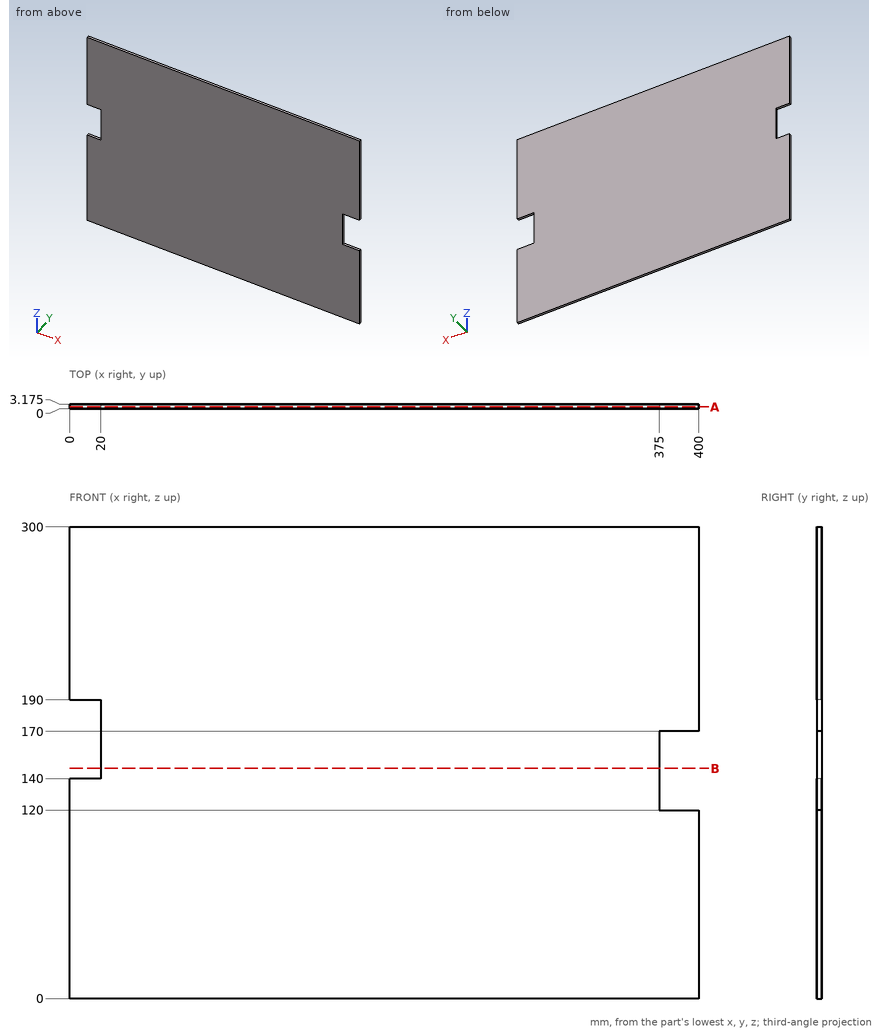
Source: three-view drawing plus pictorial views. Frame: mm from the lowest corner of the part. Give positions to 0.01 mm unless a question says otherwise; leave off trailing zeros. Order: outer loops, then holes, each group sorted by start corner. A loop starts at its lowest first (then second) coordinate and runs counter-clockwise, first axis right, second up. Notation, with made-up numbers: (77, 69) -> (130, 69) arc R24 cw to (130, 98) -> close; hole circle Ø9 at (82.5, 63.25). An arc over 180 degrees is marked (long way). Put each result on its own line as item: value.
Q1. Section A-A, the plane y = 1.4. Return loops of the section in (x, z).
Here are the results:
outline: (0, 0) -> (400, 0) -> (400, 120) -> (375, 120) -> (375, 170) -> (400, 170) -> (400, 300) -> (0, 300) -> (0, 190) -> (20, 190) -> (20, 140) -> (0, 140) -> close
Q2. Section B-B, the plane z = 146.5. Return loops of the section in (x, y) (3 decimals), then the cut area to 3 significant figures.
Here are the results:
outline: (20, 0) -> (375, 0) -> (375, 3.175) -> (20, 3.175) -> close
area: 1,130 mm^2
Q3. Material intervals for L1, parallel to Z at x = 383, y = 3.05; L2, parallel to X at y = 0.25, z = 145, sorted ascending.
Here are the results:
L1: z = 0 to 120, 170 to 300
L2: x = 20 to 375
